Here's how the part is built. I have some questions about the finished solid (model axes, mm). Coordinates: 2 decimals unless noted, no trailing zeros. Order: outer loops, then holes, each group sorted by start corner. A loop starts at its lowest first (then second) coordinate and runs counter-clockwise, first axis right, second up. Notation, with made-up numbers: (58.25, -28.75) - (86.25, -28.75) arc R21 cw to (86.25, 4.25) - close; hole circle Ø2 at (74.25, 88). An arc over 180 degrees is marked (long way). Use CSV: the item, a comma, the result in double quotes. Start each with the question number.
from build123d import *

# Parameters (mm, degrees)
SKETCH1_R                = 6.35
BOSS_EXTRUDE1_DEPTH      = 5.08
F_0_257_DIAMETER_HOLE1_D = 6.5278
CHAMFER1_SIZE            = 0.5


with BuildPart() as part:
    # Sketch1 → Boss-Extrude1 (new body)
    with BuildSketch(Plane(origin=(0, 0, 0), x_dir=(1, 0, 0), z_dir=(0, 1, 0))):
        with Locations(Location((0, 0, 0), (0, 0, 270))):
            Circle(SKETCH1_R)
    extrude(amount=BOSS_EXTRUDE1_DEPTH)

    # F (0.257) Diameter Hole1 (through all)
    with Locations(Plane(origin=(0, 5.08, 0), x_dir=(1, 0, 0), z_dir=(0, 1, 0))):
        with Locations((0, 0)):
            Hole(F_0_257_DIAMETER_HOLE1_D / 2)

    # Chamfer1
    chamfer1_edges = [part.edges().sort_by_distance(p)[0] for p in [
        (0, 0, -6.35),
        (0, 5.08, -6.35),
        (3.2639, 5.08, 0),
        (3.2639, 0, 0),
    ]]
    chamfer(chamfer1_edges, length=CHAMFER1_SIZE)


solid = part.part
Item 1: For pin 1 Ø2 at (x, z) = (-4, -4) entering from -Y; pin 2 Ø1.5 at (y, z) = (2, 1) entering from +X, each with a flat end and sliding along its axis, tell me the tip position at first contact or that it passes through.
Item 2: Suppose I cut it at C-C on y = 3.75. Write out the boundary of the cut face in (x, z), then the cut area to 3 significant figures.
Item 3: Suppose I cut it at A-A on z = 0. Write out the boundary of the cut face in (x, y).
Item 4: Please list where these lines run through material, in increasing order: line 1 along X through (y, z) = (1.65, 0); line 2 along X through (y, z) = (2.1, -1.75); line 3 along Z through (x, y) = (2, 3.05). Write a range as from..to.
Item 5: Suppose I cut it at B-B on x = 0. Write out the boundary of the cut face in (y, z), then the cut area to 3 significant figures.
Item 6: Suppose I cut it at D-D on y = 4.75. Write out the boundary of the cut face in (x, z).
Item 7: We'd pull the mould along Z, two halves only. Please class faces 1 (the cylindrical face through (-3.86, 2.51, -5.04)), 2 (the flat face through (0, 5.08, 4)), 3 (the cylindrical face through (0.708, 2.511, 3.186)): released by +Z, released by -Z, zero draft, split by the parting line, or undercut.
Here are the results:
1,pin 1,"y = 0"
1,pin 2,"x = 6.35"
2,outline,"circle Ø12.7 at (0, 0); hole circle Ø6.53 at (0, 0)"
2,area,"93.2 mm^2"
3,outline,"(-6.35, 0.5) - (-5.85, 0) - (-3.76, 0) - (-3.26, 0.5) - (-3.26, 4.58) - (-3.76, 5.08) - (-5.85, 5.08) - (-6.35, 4.58) - close; (3.26, 0.5) - (3.76, 0) - (5.85, 0) - (6.35, 0.5) - (6.35, 4.58) - (5.85, 5.08) - (3.76, 5.08) - (3.26, 4.58) - close"
4,line 1,"-6.35..-3.26, 3.26..6.35"
4,line 2,"-6.1..-2.76, 2.76..6.1"
4,line 3,"-6.03..-2.58, 2.58..6.03"
5,outline,"(0, -5.85) - (0.5, -6.35) - (4.58, -6.35) - (5.08, -5.85) - (5.08, -3.76) - (4.58, -3.26) - (0.5, -3.26) - (0, -3.76) - close; (0, 3.76) - (0.5, 3.26) - (4.58, 3.26) - (5.08, 3.76) - (5.08, 5.85) - (4.58, 6.35) - (0.5, 6.35) - (0, 5.85) - close"
5,area,"30.4 mm^2"
6,outline,"circle Ø12.36 at (0, 0); hole circle Ø6.87 at (0, 0)"
7,face 1,"split by the parting line"
7,face 2,"zero draft"
7,face 3,"undercut"
